Could you check a few things on this model? Use its own coordinates, in mm. Give positions to 0.01 mm unless a question says otherwise; leave off trailing zeros. Loops run counter-clockwise (first coordinate to the right, second up) from the corner with the lowest first, then second, coordinate; pieces in that order, holes last. Notation, with made-up numbers: (-21, 84) -> (-3, 84) arc R29 ccw to (-3, 122) -> close; hole circle Ø11 at (75.5, 49.25). An arc over 180 degrees is marked (long way). Put each result on its own line as item: value.
```python
from build123d import *

# Parameters (mm, degrees)
SKETCH_R  = 1.627
PAD_DEPTH = 1.8542


with BuildPart() as part:
    # Sketch (on Face16 of Binder001) → Pad (new body)
    with BuildSketch(Plane.XZ.offset(-127.2271)):
        with BuildLine():
            Line((0, -23.379), (-6.8772, -23.379))
            ThreePointArc((-6.8772, -23.379), (-7.725728, -23.730472), (-8.0772, -24.579))
            Line((-8.0772, -24.579), (-8.0772, -87.921))
            ThreePointArc((-8.0772, -87.921), (-7.725728, -88.769528), (-6.8772, -89.121))
            Line((-6.8772, -89.121), (0, -89.121))
            ThreePointArc((1.2, -90.321), (0.848528, -89.472472), (0, -89.121))
            Line((1.2, -90.321), (1.2, -114.1729))
            ThreePointArc((1.2, -114.1729), (1.551472, -115.021428), (2.4, -115.3729))
            Line((2.4, -115.3729), (72.679, -115.3729))
            ThreePointArc((73.879, -116.5729), (73.527528, -115.724372), (72.679, -115.3729))
            Line((73.879, -116.5729), (73.879, -118.4271))
            ThreePointArc((73.879, -118.4271), (74.230472, -119.275628), (75.079, -119.6271))
            Line((75.079, -119.6271), (138.421, -119.6271))
            ThreePointArc((138.421, -119.6271), (139.269528, -119.275628), (139.621, -118.4271))
            Line((139.621, -118.4271), (139.621, -116.5729))
            ThreePointArc((140.821, -115.3729), (139.972472, -115.724372), (139.621, -116.5729))
            Line((140.821, -115.3729), (286.179, -115.3729))
            ThreePointArc((287.379, -116.5729), (287.027528, -115.724372), (286.179, -115.3729))
            Line((287.379, -116.5729), (287.379, -118.4271))
            ThreePointArc((287.379, -118.4271), (287.730472, -119.275628), (288.579, -119.6271))
            Line((288.579, -119.6271), (351.921, -119.6271))
            ThreePointArc((351.921, -119.6271), (352.769528, -119.275628), (353.121, -118.4271))
            Line((353.121, -118.4271), (353.121, -116.5729))
            ThreePointArc((354.321, -115.3729), (353.472472, -115.724372), (353.121, -116.5729))
            Line((354.321, -115.3729), (424.6, -115.3729))
            ThreePointArc((424.6, -115.3729), (425.448528, -115.021428), (425.8, -114.1729))
            Line((425.8, -114.1729), (425.8, -90.321))
            ThreePointArc((427, -89.121), (426.151472, -89.472472), (425.8, -90.321))
            Line((427, -89.121), (433.8772, -89.121))
            ThreePointArc((433.8772, -89.121), (434.725728, -88.769528), (435.0772, -87.921))
            Line((435.0772, -87.921), (435.0772, -24.579))
            ThreePointArc((435.0772, -24.579), (434.725728, -23.730472), (433.8772, -23.379))
            Line((433.8772, -23.379), (427, -23.379))
            ThreePointArc((425.8, -22.179), (426.151472, -23.027528), (427, -23.379))
            Line((425.8, -22.179), (425.8, 1.6729))
            ThreePointArc((425.8, 1.6729), (425.448528, 2.521428), (424.6, 2.8729))
            Line((424.6, 2.8729), (354.321, 2.8729))
            ThreePointArc((353.121, 4.0729), (353.472472, 3.224372), (354.321, 2.8729))
            Line((353.121, 4.0729), (353.121, 5.9271))
            ThreePointArc((353.121, 5.9271), (352.769528, 6.775628), (351.921, 7.1271))
            Line((351.921, 7.1271), (288.579, 7.1271))
            ThreePointArc((288.579, 7.1271), (287.730472, 6.775628), (287.379, 5.9271))
            Line((287.379, 5.9271), (287.379, 4.0729))
            ThreePointArc((286.179, 2.8729), (287.027528, 3.224372), (287.379, 4.0729))
            Line((286.179, 2.8729), (227.82595, 2.8729))
            ThreePointArc((227.82595, 2.8729), (226.977422, 2.521428), (226.62595, 1.6729))
            Line((226.62595, 1.6729), (226.62595, -22.179))
            ThreePointArc((225.42595, -23.379), (226.274478, -23.027528), (226.62595, -22.179))
            Line((225.42595, -23.379), (201.57405, -23.379))
            ThreePointArc((200.37405, -22.179), (200.725522, -23.027528), (201.57405, -23.379))
            Line((200.37405, -22.179), (200.37405, 1.6729))
            ThreePointArc((200.37405, 1.6729), (200.022578, 2.521428), (199.17405, 2.8729))
            Line((199.17405, 2.8729), (140.821, 2.8729))
            ThreePointArc((139.621, 4.0729), (139.972472, 3.224372), (140.821, 2.8729))
            Line((139.621, 4.0729), (139.621, 5.9271))
            ThreePointArc((139.621, 5.9271), (139.269528, 6.775628), (138.421, 7.1271))
            Line((138.421, 7.1271), (75.079, 7.1271))
            ThreePointArc((75.079, 7.1271), (74.230472, 6.775628), (73.879, 5.9271))
            Line((73.879, 5.9271), (73.879, 4.0729))
            ThreePointArc((72.679, 2.8729), (73.527528, 3.224372), (73.879, 4.0729))
            Line((72.679, 2.8729), (2.4, 2.8729))
            ThreePointArc((2.4, 2.8729), (1.551472, 2.521428), (1.2, 1.6729))
            Line((1.2, 1.6729), (1.2, -22.179))
            ThreePointArc((0, -23.379), (0.848528, -23.027528), (1.2, -22.179))
        make_face()
        with Locations((194.45, -74.03)):
            Circle(SKETCH_R, mode=Mode.SUBTRACT)
        with Locations((232.55, -74.03)):
            Circle(SKETCH_R, mode=Mode.SUBTRACT)
        with Locations((283.35, -74.03)):
            Circle(SKETCH_R, mode=Mode.SUBTRACT)
        with Locations((334.15, -74.03)):
            Circle(SKETCH_R, mode=Mode.SUBTRACT)
        with Locations((384.95, -74.03)):
            Circle(SKETCH_R, mode=Mode.SUBTRACT)
        with Locations((143.65, -74.03)):
            Circle(SKETCH_R, mode=Mode.SUBTRACT)
        with Locations((92.85, -74.03)):
            Circle(SKETCH_R, mode=Mode.SUBTRACT)
        with Locations((42.05, -74.03)):
            Circle(SKETCH_R, mode=Mode.SUBTRACT)
        with Locations((106.75, -2.0081)):
            Circle(SKETCH_R, mode=Mode.SUBTRACT)
        with Locations((106.75, -110.4919)):
            Circle(SKETCH_R, mode=Mode.SUBTRACT)
        with Locations((320.25, -110.4919)):
            Circle(SKETCH_R, mode=Mode.SUBTRACT)
        with Locations((320.25, -2.0081)):
            Circle(SKETCH_R, mode=Mode.SUBTRACT)
        with BuildLine():
            ThreePointArc((-1.7272, -48.25), (-3.4417, -46.5355), (-5.1562, -48.25))
            Line((-5.1562, -48.25), (-5.1562, -64.25))
            ThreePointArc((-5.1562, -64.25), (-3.4417, -65.9645), (-1.7272, -64.25))
            Line((-1.7272, -48.25), (-1.7272, -64.25))
        make_face(mode=Mode.SUBTRACT)
        with BuildLine():
            ThreePointArc((432.1562, -48.25), (430.4417, -46.5355), (428.7272, -48.25))
            Line((428.7272, -48.25), (428.7272, -64.25))
            ThreePointArc((428.7272, -64.25), (430.4417, -65.9645), (432.1562, -64.25))
            Line((432.1562, -48.25), (432.1562, -64.25))
        make_face(mode=Mode.SUBTRACT)
    extrude(amount=PAD_DEPTH)


solid = part.part
```
1. If we section it at A-A (x = 205.5): List the corners of the cut face in (y, z) for me.
Recorded:
outline: (125.37, -115.37) -> (127.23, -115.37) -> (127.23, -23.38) -> (125.37, -23.38) -> close
2. I need wall thicknesses on line 1 (Z direction, x = 320.25, y = 125.85); line 2 (X direction, y = 126.4, z = -57); line 3 (X direction, y = 126.6, z = -64.5). Which ranges of each line are inside material? Lowest first, please.
Recorded:
line 1: z = -119.63 to -112.12, -108.86 to -3.64, -0.38 to 7.13
line 2: x = -8.08 to -5.16, -1.73 to 428.73, 432.16 to 435.08
line 3: x = -8.08 to -5.14, -1.75 to 428.75, 432.14 to 435.08
3. I'm going to push flat-ended pins straight in: pin 1 (0.9 mm diameter, centred on y = 126, z = 5, fed in from -X); pin 2 (0.9 mm diameter, centred on x = -2.5, y = 126, fed in from +Z); pin 3 (2.5 mm diameter, centred on x = 283.35, z = -74.03, fed in from +Y); pin 4 (0.9 mm diameter, centred on y = 126, z = -9.5, fed in from +X). Where does each tip first touch, or does it pass through?
Recorded:
pin 1: stops at x = 73.88
pin 2: stops at z = -23.38
pin 3: passes through
pin 4: stops at x = 425.8
4. If we section it at C-C (x = 401): List the corners of the cut face in (y, z) for me, then the cut area to 3 significant figures.
Recorded:
outline: (125.37, -115.37) -> (127.23, -115.37) -> (127.23, 2.87) -> (125.37, 2.87) -> close
area: 219 mm^2
5. If we section it at B-B (y = 125.75): Count the separate pieces of the cut face and the enclosed holes in it, then the cut area to 3 significant figures.
Recorded:
separate pieces: 1
enclosed holes: 14
area: 51,600 mm^2
